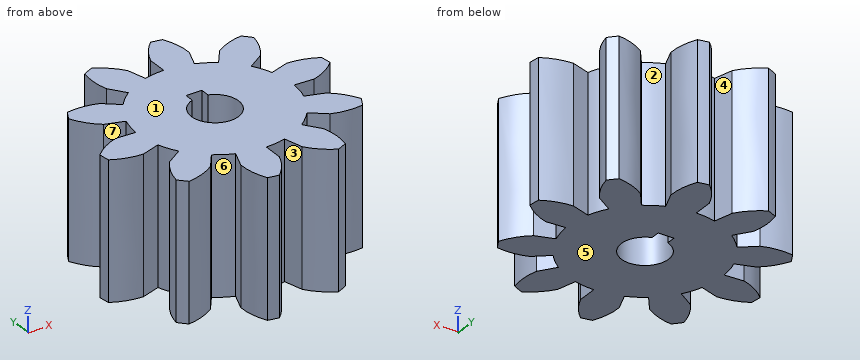
```python
from build123d import *

# Parameters (mm, degrees)
BOSS_EXTRUDE1_DEPTH = 43.5
CIRPATTERN1_COUNT   = 10
SKETCH2_R           = 7.5
CUT_EXTRUDE1_DEPTH  = 70.959609915
SKETCH3_W           = 5
SKETCH3_H           = 5
CUT_EXTRUDE2_DEPTH  = 70.959609915


with BuildPart() as part:
    # Sketch1 → Boss-Extrude1 (new body)
    with BuildSketch(Plane.XY):
        with BuildLine():
            add(Edge.make_bspline(
                [(0, 30.535), (1.094025697, 33.738879921), (2.960368297, 36.423385517), (5.329249796, 38.634170065)],
                knots=[0, 0, 0, 0, 0.089409401, 0.089409401, 0.089409401, 0.089409401], degree=3))
            Line((0, 30.535), (0, 24.375))
            ThreePointArc((0, 24.375), (-4.413773565, -23.972050974), (8.681616812, 22.776526393))
            Line((8.681616812, 22.776526393), (10.875617204, 28.532563422))
            add(Edge.make_bspline(
                [(10.875617204, 28.532563422), (10.994458338, 31.915995933), (10.206644899, 35.089189117), (8.780523558, 37.998715847)],
                knots=[0, 0, 0, 0, 0.089409401, 0.089409401, 0.089409401, 0.089409401], degree=3))
            ThreePointArc((8.780523558, 37.998715847), (7.062037704, 38.355281559), (5.329249796, 38.634170065))
        make_face()
    boss_extrude1 = extrude(amount=BOSS_EXTRUDE1_DEPTH)

    # CirPattern1: Boss-Extrude1 ×10 about axis
    cirpattern1_axis = Axis((0, 0, 0), (0, 0, -1))
    for i in range(1, CIRPATTERN1_COUNT):
        add(boss_extrude1.rotate(cirpattern1_axis, i * 360 / CIRPATTERN1_COUNT))

    # Sketch2 → Cut-Extrude1 (cut, through all)
    with BuildSketch(Plane.XY.offset(43.5)):
        Circle(SKETCH2_R)
    extrude(amount=-CUT_EXTRUDE1_DEPTH, mode=Mode.SUBTRACT)

    # Sketch3 → Cut-Extrude2 (cut, through all)
    with BuildSketch(Plane.XY.offset(43.5)):
        with Locations((0, 7.5)):
            Rectangle(SKETCH3_W, SKETCH3_H)
    extrude(amount=-CUT_EXTRUDE2_DEPTH, mode=Mode.SUBTRACT)


solid = part.part
```
Here's how the part is built. I have some questions about the finished solid (model axes, mm). Face numbers are marked on the shaded views. A direction names the side the tool comes from. Give positions to 0.01 mm unless a question says otherwise; leave off trailing zeros. Answer as a JSON object with one key per item and string values. Group by question number.
Item 1: For P1, Ø4, axis at x = 0, z = 25.5, coming from the -Y side; P2, Ø1.5, axis at y = 8.5, z = 12, coming from the +X side; P3, Ø8, axis at x = 15.5, z = 36.5, coming from the -Y side; P4, Ø13.5, axis at x = 0, y = 0, coming from the +Z side, each with a flat end and sliding along its axis, tell me the tip position at first contact or that it passes through.
Item 2: Which directions (+Z, -Z, +X, -X, +Y, -Y) give clear straight access to the entire face, cutting with the end or side of a thin tool? Please do the marked faces 4, 5, 6 and 7.
Item 3: Please list where these lines run through material, in increasing order: probe 1 along Y at (x, z) = (26.5, 32); probe 2 along Y at (x, z) = (-26.5, 35); probe 3 along Y at (x, z) = (4.5, 17).
Item 4: If we mould it in two halves opening along Y, with no side actions, what happens to the marked faces 1, 2 and 3? For each: pulls with the +Y half, pulls with the -Y half, needs draft (parallel to the pull), parting line crosses it, or undercut.
Result set:
{
 "1": {"P1": "y = -34.67", "P2": "x = 36.62", "P3": "y = -35.9", "P4": "through"},
 "2": {"face 4": "+Z, -Z, +Y", "face 5": "-Z, +X, -X, +Y, -Y", "face 6": "+Z, -Z", "face 7": "+Z, -Z, -X"},
 "3": {"probe 1": "-19.93 to -8.61, -1.33 to 8.61, 17.99 to 28.05", "probe 2": "-28.05 to -17.99, -8.61 to 1.33, 8.61 to 19.93", "probe 3": "-23.96 to -6, 6 to 37.82"},
 "4": {"face 1": "needs draft", "face 2": "undercut", "face 3": "pulls with the -Y half"}
}
